from build123d import *

# Parameters (mm, degrees)
F0_R        = 10
F1_DEPTH    = 4
F2_R        = 0.5
F3_T1_DEPTH = 40.2304088715
F4_T1_DEPTH = 4
F5_SIZE     = 20
F6_R        = 20


# Not quite as in the source:
# - a fillet or chamfer that OpenCascade refuses, or shapes differently, is made with other operations: its cross-section is extruded or revolved along the edge and cut away or added


with BuildPart() as f1:
    # F0 (on Top) → F1 (new body)
    with BuildSketch(Plane.XY):
        with BuildLine():
            Line((50, 20.5837816147), (50, 12.9642039537))
            Line((50, 12.9642039537), (-16.1380209029, 9.3462867662))
            Line((-16.1380209029, 9.3462867662), (-50, 0))
            Line((-50, 0), (-16.1380209029, -9.3462867662))
            Line((-16.1380209029, -9.3462867662), (50, -12.9642039537))
            Line((50, -12.9642039537), (50, -22.5))
            Line((50, -22.5), (55, -22.5))
            ThreePointArc((55, -22.5), (56.5936558821, -15.0125045804), (62.1990375221, -9.7988663689))
            ThreePointArc((62.1990375221, -9.7988663689), (98.7587484272, -9.3015269429), (135, -14.1421356237))
            ThreePointArc((135, -14.1421356237), (155, 0), (135, 14.1421356237))
            ThreePointArc((135, 14.1421356237), (98.7587484272, 9.3015269429), (62.1990375221, 9.7988663689))
            ThreePointArc((62.1990375221, 9.7988663689), (57.1204966078, 14.2040620862), (55, 20.5837816147))
            Line((55, 20.5837816147), (50, 20.5837816147))
        make_face()
        with BuildLine():
            ThreePointArc((62.1990375221, -4.8343795659), (60.2509894701, 0), (62.1990375221, 4.8343795659))
            ThreePointArc((62.1990375221, 4.8343795659), (94.7590329876, 4.3577585856), (127.1470964452, 7.7332315503))
            ThreePointArc((127.1470964452, 7.7332315503), (125, 0), (127.1470964452, -7.7332315503))
            ThreePointArc((127.1470964452, -7.7332315503), (94.7590329876, -4.3577585856), (62.1990375221, -4.8343795659))
        make_face(mode=Mode.SUBTRACT)
        with Locations((140, 0)):
            Circle(F0_R, mode=Mode.SUBTRACT)
    extrude(amount=F1_DEPTH)

    # F2
    f2_edges = [f1.edges().sort_by_distance(p)[0] for p in [
        (127.147096, 7.733232, 2),
        (127.147096, -7.733232, 2),
    ]]
    fillet(f2_edges, radius=F2_R)

    # F3: fillet of radius 2 on 1 edges, made by hand

    # F3_s2 → F3_t1 (cut)
    with BuildSketch(Plane.XY.offset(-18.1152044358)):
        with BuildLine():
            ThreePointArc((-43.0150978282, 1.9279114946), (-44.4829725902, 0), (-43.0150978282, -1.9279114946))
            Line((-43.0150978282, -1.9279114946), (-50, 0))
            Line((-50, 0), (-43.0150978282, 1.9279114946))
        make_face()
    extrude(amount=F3_T1_DEPTH, mode=Mode.SUBTRACT)

    # F4: fillet of radius 20 on 2 edges, made by hand

    # F4_s2 → F4_t1 (join)
    with BuildSketch(Plane.XY):
        with BuildLine():
            ThreePointArc((34.7404872131, 12.1294699712), (43.3406010629, 14.6051902372), (50, 20.5837816147))
            Line((50, 20.5837816147), (50, 12.9642039537))
            Line((50, 12.9642039537), (34.7404872131, 12.1294699712))
        make_face()
        with BuildLine():
            ThreePointArc((50, -22.5), (43.1146209861, -15.1332813357), (33.5101814977, -12.0621691338))
            Line((33.5101814977, -12.0621691338), (50, -12.9642039537))
            Line((50, -12.9642039537), (50, -22.5))
        make_face()
    extrude(amount=F4_T1_DEPTH)

    # F5
    f5_edges = [f1.edges().sort_by_distance(p)[0] for p in [
        (-16.138021, -9.346287, 2),
        (-16.138021, 9.346287, 2),
    ]]
    chamfer(f5_edges, length=F5_SIZE)

    # F6
    f6_edges = [f1.edges().sort_by_distance(p)[0] for p in [
        (-35.417136, 4.025034, 2),
        (-35.417136, -4.025034, 2),
    ]]
    fillet(f6_edges, radius=F6_R)


solid = f1.part
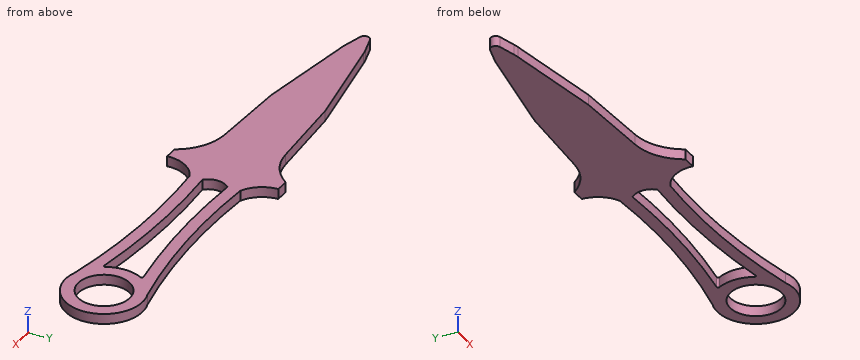
Part model, mm, in its own coordinate system. Coordinates: 2 decimals unless noted, no trailing zeros. Write each loop counter-clockwise with the first axis right and the second up, starting at its lowest first coordinate (ties: lowest second). Pieces come first, ordered by that corner, then holes. Notation, with made-up numbers: M 17,53 L 51,53 A16 cw 51,61 Z; hole C 63,11 d5. An arc over 180 degrees is marked long. Return JSON: item names as keys, results as strings.
1. Flat gauge pins, fed straight in: pin 1 Ø2 at (y, z) = (-15.5, 2.5) entering from -X; pin 2 Ø1 at (x, z) = (-15, 3) entering from -Y; pin 3 Ø18 at (x, y) = (140, 0) entering from -Z; pin 4 Ø1.5 at (y, z) = (-3.5, 3) entering from +X. Where does each tip first touch, or does it go through?
Determined:
{"pin 1": "x = 42.04", "pin 2": "y = -7.44", "pin 3": "through", "pin 4": "x = 154.75"}
2. Saw through at A-A, the plane y = 0. Write the cut outline in (x, z), then the cut area to 3 significant figures.
Determined:
{"outline": "M -44.48,0 L 60.25,0 L 60.25,4 L -44.48,4 Z; M 125,0 L 130,0 L 130,4 L 125,4 Z; M 150,0 L 155,0 L 155,4 L 150,4 Z", "area": "459 mm²"}
3. Probe L1, parallel to X at y = 1.5, z = 0.2; L2, parallel to Y at x = 140, z = 2.9; L3, parallel to X at y = 1, z = 2.85. List the from-to ranges inside material, lowest first.
Determined:
{"L1": "-43.81 to 60.41, 125.08 to 130.11, 149.89 to 154.92", "L2": "-15 to -10, 10 to 15", "L3": "-44.22 to 60.32, 125.03 to 130.05, 149.95 to 154.97"}
4. Saw through at D-D, the plane x = 26. Write the cut outline in (y, z), then the cut area to 3 significant figures.
Determined:
{"outline": "M -11.65,0 L 11.65,0 L 11.65,4 L -11.65,4 Z", "area": "93.2 mm²"}
5. Saw through at C-C, the plane z = 0.75. Count the separate pieces of the cut face and the enclosed holes in it, then the cut area to 3 significant figures.
Determined:
{"separate pieces": "1", "enclosed holes": "2", "area": "3,210 mm²"}
6. Saw through at B-B, the plane x = 140. Write the cut outline in (y, z).
Determined:
{"outline": "M -15,0 L -10,0 L -10,4 L -15,4 Z; M 10,0 L 15,0 L 15,4 L 10,4 Z"}
